```python
from build123d import *

# Parameters (mm, degrees)
BOSS_EXTRUDE1_DEPTH = 35
FILLET1_R           = 5
CHAMFER1_SIZE       = 1
SKETCH2_W           = 35
SKETCH2_H           = 20
BOSS_EXTRUDE2_DEPTH = 30
FILLET2_R           = 2
SKETCH3_W           = 35
SKETCH3_H           = 20
BOSS_EXTRUDE3_DEPTH = 30
FILLET3_R           = 2
FILLET4_R           = 2
SKETCH4_R           = 5.25
CUT_EXTRUDE1_DEPTH  = 20


with BuildPart() as part:
    # Sketch1 → Boss-Extrude1 (new body)
    with BuildSketch(Plane.XY):
        with BuildLine():
            Line((0, 0), (-200, 0))
            Line((-200, 0), (-200, 66.385933837))
            ThreePointArc((-200, 66.385933837), (-100, 35), (0, 66.385933837))
            Line((0, 66.385933837), (0, 0))
        make_face()
        with BuildLine():
            ThreePointArc((-184.216990788, 43.037433948), (-100, 23), (-15.783009212, 43.037433948))
            ThreePointArc((-15.783009212, 43.037433948), (-10.141543229, 41.178977178), (-12, 35.537511195))
            ThreePointArc((-12, 35.537511195), (-100, 14.6), (-188, 35.537511195))
            ThreePointArc((-188, 35.537511195), (-189.858456771, 41.178977178), (-184.216990788, 43.037433948))
        make_face(mode=Mode.SUBTRACT)
    extrude(amount=BOSS_EXTRUDE1_DEPTH)

    # Fillet1
    fillet1_edges = [part.edges().sort_by_distance(p)[0] for p in [
        (-200, 66.385933837, 17.5),
        (0, 66.385933837, 17.5),
    ]]
    fillet(fillet1_edges, radius=FILLET1_R)

    # Chamfer1
    chamfer1_edges = [part.edges().sort_by_distance(p)[0] for p in [
        (-189.858456771, 41.178977178, 0),
        (-100, 14.6, 0),
        (-10.141543229, 41.178977178, 0),
        (-100, 23, 0),
        (-189.858456771, 41.178977178, 35),
        (-100, 14.6, 35),
        (-10.141543229, 41.178977178, 35),
        (-100, 23, 35),
    ]]
    chamfer(chamfer1_edges, length=CHAMFER1_SIZE)

    # Sketch2 → Boss-Extrude2 (add)
    with BuildSketch(Plane(origin=(0, 0, 0), x_dir=(0, 0, -1), z_dir=(1, 0, 0))):
        with Locations((-17.5, 10)):
            Rectangle(SKETCH2_W, SKETCH2_H)
    extrude(amount=BOSS_EXTRUDE2_DEPTH)

    # Fillet2
    fillet2_edges = [part.edges().sort_by_distance(p)[0] for p in [
        (0, 20, 17.5),
    ]]
    fillet(fillet2_edges, radius=FILLET2_R)

    # Sketch3 → Boss-Extrude3 (add)
    with BuildSketch(Plane.ZY.offset(200)):
        with Locations((17.5, 10)):
            Rectangle(SKETCH3_W, SKETCH3_H)
    extrude(amount=BOSS_EXTRUDE3_DEPTH)

    # Fillet3
    fillet3_edges = [part.edges().sort_by_distance(p)[0] for p in [
        (-200, 20, 17.5),
    ]]
    fillet(fillet3_edges, radius=FILLET3_R)

    # Fillet4
    fillet4_edges = [part.edges().sort_by_distance(p)[0] for p in [
        (30, 10, 35),
        (30, 10, 0),
        (-230, 10, 0),
        (-230, 10, 35),
    ]]
    fillet(fillet4_edges, radius=FILLET4_R)

    # Sketch4 → Cut-Extrude1 (cut)
    with BuildSketch(Plane(origin=(0, 20, 0), x_dir=(1, 0, 0), z_dir=(0, 1, 0))):
        with Locations(Location((-215, -17.5, 0), (0, 0, 270))):
            Circle(SKETCH4_R)
        with Locations(Location((15, -17.5, 0), (0, 0, 270))):
            Circle(SKETCH4_R)
    extrude(amount=-CUT_EXTRUDE1_DEPTH, mode=Mode.SUBTRACT)


solid = part.part
```
Model file for the job. Use its own axes, mm. A direction names the side the tool comes from. Round coordinates to 2 decimals unless told otherwise and drop trailing zeros. Write each loop counter-clockwise with the first axis right and the second up, starting at its lowest first coordinate (ties: lowest second). Pieces come first, ordered by that corner, then holes. Notation, with made-up numbers: (34, -33) - (71, -33) arc R18 ccw to (71, -11) - close; hole circle Ø3 at (55, 48). An arc over 180 degrees is marked (long way). Use CSV: the item, a comma, the result in double quotes. Start each with the question number.
Item 1: Two-plate mould, pull along Z, no slides. Class faces 1 (the face through (0, 40, 17)), 2 (the face through (15.231, 10.14, 12.255)), 3 (the face through (-98, 31, 0)): released by +Z, released by -Z, zero draft, split by the parting line, or undercut.
Item 2: Drill centre lines: L1, parallel to X at y = 5.25, z = 17.5; L2, parallel to Y at x = -116.5, z = 18; L3, parallel to Y at x = -204.5, z = 4. Where is each one in solid material? Low to high. Write a range as [from, to].
Item 3: Band-saw the part on D-D (y = 26). State how many separate pieces and enclosed holes the cut face has, and give its area (3 significant figures).
Item 4: Tool access for faces 4 (the face through (-200, 39, 17)), 5 (the face through (-218.19, 10.14, 13.33)), 6 (the face through (-98.722, 14.604, 17.269)), 7 (the face through (19, 20, 22)): list every direction of +Z, -Z, +X, -X, +Y, -Y with a clear straight run to the whole face (end or side of a thin tool).
Item 5: Band-saw the part on B-B (z = 17.5). Write the cut outline in (x, y).
Item 6: Pin check, flat tips, straight feed: P1, Ø6, axis at y = 25, z = 12, coming from the -X side; P2, Ø10, axis at y = 27.5, z = 22.5, coming from the +X side; P3, Ø6, axis at x = -37, z = 11.5, coming from the +Y side; P4, Ø9.5, axis at x = 15, z = 17.5, coming from the +Y side. Stop position of each tip, or through.
Item 7: Band-saw the part on C-C (y = 48.5). Write the cut outline in (x, z), and give its area (3 significant figures).
Item 8: Band-saw the part on A-A (x = 15). Write the cut outline in (y, z).
Checked values:
1,face 1,"zero draft"
1,face 2,"undercut"
1,face 3,"released by -Z"
2,L1,"x = [-230, -220.25], [-209.75, 9.75], [20.25, 30]"
2,L2,"y = [0, 15.3], [23.73, 35.78]"
2,L3,"y = [0, 20]"
3,separate pieces,"3"
3,enclosed holes,"0"
3,area,"4,710 mm²"
4,face 4,"+Z, -Z, -X, +Y"
4,face 5,"+Y, -Y"
4,face 6,"+Z, -Z"
4,face 7,"+Z, -Z, +X, +Y"
5,outline,"(-230, 0) - (-220.25, 0) - (-220.25, 20) - (-230, 20) - close; (-209.75, 0) - (9.75, 0) - (9.75, 20) - (2, 20) arc R2 cw to (0, 22) - (0, 57.11) arc R5 ccw to (-7.64, 61.36) arc R175 cw to (-192.36, 61.36) arc R5 ccw to (-200, 57.11) - (-200, 22) arc R2 cw to (-202, 20) - (-209.75, 20) - close; (20.25, 0) - (30, 0) - (30, 20) - (20.25, 20) - close; hole (-188, 35.54) arc R195.4 ccw to (-12, 35.54) arc R4.2 ccw to (-15.78, 43.04) arc R187 cw to (-184.22, 43.04) arc R4.2 ccw to start"
6,P1,"stops at x = -200"
6,P2,"stops at x = 0"
6,P3,"stops at y = 47.92"
6,P4,"passes through"
7,outline,"(-200, 0) - (-167.4, 0) - (-167.4, 35) - (-200, 35) - close; (-32.6, 0) - (0, 0) - (0, 35) - (-32.6, 35) - close"
7,area,"2,280 mm²"
8,outline,"(0, 0) - (20, 0) - (20, 12.25) - (0, 12.25) - close; (0, 22.75) - (20, 22.75) - (20, 35) - (0, 35) - close"
